```python
from build123d import *

# Parameters (mm, degrees)
BOSS_EXTRUDE1_DEPTH = 3
SKETCH1_W           = 20
SKETCH1_H           = 3
BOSS_EXTRUDE2_DEPTH = 2
SKETCH2_W           = 20
SKETCH2_H           = 3
BOSS_EXTRUDE3_DEPTH = 2
CUT_EXTRUDE4_DEPTH  = 44
SKETCH4_R           = 0.75
CUT_EXTRUDE5_DEPTH  = 16
CUT_EXTRUDE6_DEPTH  = 16


with BuildPart() as part:
    # Model → Boss-Extrude1 (new body)
    with BuildSketch(Plane.XY):
        Polygon((70.216761418, 10.802709547), (53.276888396, 10.802709547), (53.276888396, 9.302709547), (33.276888396, 9.302709547), (33.276888396, 10.802709547), (16.337015373, 10.802709547), (16.337015373, 50.802709547), (33.276888396, 50.802709547), (33.276888396, 52.283127555), (53.276888396, 52.283127555), (53.276888396, 50.802709547), (70.216761418, 50.802709547), align=None)
    extrude(amount=BOSS_EXTRUDE1_DEPTH)

    # Sketch1 → Boss-Extrude2 (add)
    with BuildSketch(Plane.XZ.offset(-9.302709547)):
        with Locations((43.276888396, 1.5)):
            Rectangle(SKETCH1_W, SKETCH1_H)
    extrude(amount=BOSS_EXTRUDE2_DEPTH)

    # Sketch2 → Boss-Extrude3 (add)
    with BuildSketch(Plane(origin=(0, 52.283127555, 0), x_dir=(1, 0, 0), z_dir=(0, 1, 0))):
        with Locations((43.276888396, -1.5)):
            Rectangle(SKETCH2_W, SKETCH2_H)
    extrude(amount=BOSS_EXTRUDE3_DEPTH)

    # Sketch3 → Cut-Extrude4 (cut)
    with BuildSketch(Plane(origin=(0, 50.802709547, 0), x_dir=(1, 0, 0), z_dir=(0, 1, 0))):
        Polygon((70.216761418, 0), (69.716761418, 0), (70.216761418, -3), align=None)
        Polygon((16.337015373, -3), (16.337015373, 0), (16.837015373, 0), align=None)
    extrude(amount=-CUT_EXTRUDE4_DEPTH, mode=Mode.SUBTRACT)

    # Sketch4 → Cut-Extrude5 (cut)
    with BuildSketch(Plane.XY.offset(3)):
        with Locations((22.776888396, 39.218622605)):
            Circle(SKETCH4_R)
        with Locations((22.776888396, 22.718622605)):
            Circle(SKETCH4_R)
        with Locations(Location((63.776888396, 22.718622605, 0), (0, 0, 180))):
            Circle(SKETCH4_R)
        with Locations(Location((63.776888396, 39.218622605, 0), (0, 0, 180))):
            Circle(SKETCH4_R)
    extrude(amount=-CUT_EXTRUDE5_DEPTH, mode=Mode.SUBTRACT)

    # Sketch5 → Cut-Extrude6 (cut)
    with BuildSketch(Plane.XY.offset(3)):
        with BuildLine():
            Line((32.633411635, 20.459880451), (53.935807441, 20.459880451))
            ThreePointArc((53.935807441, 20.459880451), (56.222748266, 18.172939626), (53.935807441, 15.885998802))
            Line((53.935807441, 15.885998802), (32.633411635, 15.885998802))
            ThreePointArc((32.633411635, 15.885998802), (30.34647081, 18.172939626), (32.633411635, 20.459880451))
        make_face()
    extrude(amount=-CUT_EXTRUDE6_DEPTH, mode=Mode.SUBTRACT)


solid = part.part
```
Here's how the part is built. I have some questions about the finished solid (model axes, mm). A direction names the side the tool comes from. Round coordinates to 2 decimals unless told otherwise and drop trailing zeros. Write each loop counter-clockwise with the first axis right and the second up, starting at its lowest first coordinate (ties: lowest second). Pieces come first, ordered by that corner, then holes.
Q1. Which directions (+Z, -Z, +X, -X, +Y, -Y) give clear straight access to the entire face, cutting with the end or side of a thin tool? Please do faces 4 (the flat face through (33.277, 9, 1)), 5 (the cylindrical face through (56.222, 18.223, 1.521)), 6 (the flat face through (62, 10.803, 1)), 7 (the flat face through (62, 50.803, 1)).
Q2. If we section it at B-B on x = 55: Write out the boundary of the cut face in (y, z), plus the area to 3 significant figures.
Q3. If we section it at C-C on x = 29: Write out the boundary of the cut face in (y, z), plus the area to 3 significant figures.
Q4. Will these pins go through, and if not, where does the flat tip stop? P1, Ø1.5, axis at y = 53, z = 2, coming from the +X side; P2, Ø1.5, axis at x = 61.5, z = 2.5, coming from the -Y side; P3, Ø1, axis at y = 21, z = 2, coming from the +X side.
Q5. If we mould it in two halves opening along Y, with no side actions, what happens to faces 1 (the flat face through (33.277, 53, 2)), 2 (the flat face through (43, 15.886, 2)), 3 (the flat face through (25, 50.803, 1))? For each: +Y half, -Y half, draft (parallel to the pull), parting line (faces both ways), or undercut.
Q6. Please list where these lines run through material, in increasing order: probe 1 along Y at (x, z) = (46.5, 0.25); probe 2 along Y at (x, z) = (28.5, 0.6); probe 3 along Y at (x, z) = (64, 1).
Q7. If we section it at A-A on z = 0.55: Write out the boundary of the cut face in (x, y), plus the area to 3 significant figures.
Answer below:
1. face 4: +Z, -Z, -X, -Y
1. face 5: +Z, -Z
1. face 6: +Z, -Z, +X, -Y
1. face 7: +Z, -Z, +X, +Y
2. outline: (10.8, 0) - (16.15, 0) - (16.15, 3) - (10.8, 3) - close; (20.2, 0) - (50.8, 0) - (50.8, 3) - (20.2, 3) - close
2. area: 108 mm2
3. outline: (10.8, 0) - (50.8, 0) - (50.8, 3) - (10.8, 3) - close
3. area: 120 mm2
4. P1: stops at x = 53.28
4. P2: stops at y = 10.8
4. P3: stops at x = 70.13
5. face 1: draft
5. face 2: undercut
5. face 3: +Y half
6. probe 1: y = 7.3 to 15.89, 20.46 to 54.28
6. probe 2: y = 10.8 to 50.8
6. probe 3: y = 10.8 to 22, 23.43 to 38.5, 39.93 to 50.8
7. outline: (16.75, 10.8) - (33.28, 10.8) - (33.28, 7.3) - (53.28, 7.3) - (53.28, 10.8) - (69.81, 10.8) - (69.81, 50.8) - (53.28, 50.8) - (53.28, 54.28) - (33.28, 54.28) - (33.28, 50.8) - (16.75, 50.8) - close; hole circle Ø1.5 at (22.78, 22.72); hole circle Ø1.5 at (22.78, 39.22); hole (32.63, 15.89) - (53.94, 15.89) arc R2.29 ccw to (53.94, 20.46) - (32.63, 20.46) arc R2.29 ccw to start; hole circle Ø1.5 at (63.78, 22.72); hole circle Ø1.5 at (63.78, 39.22)
7. area: 2,140 mm2
